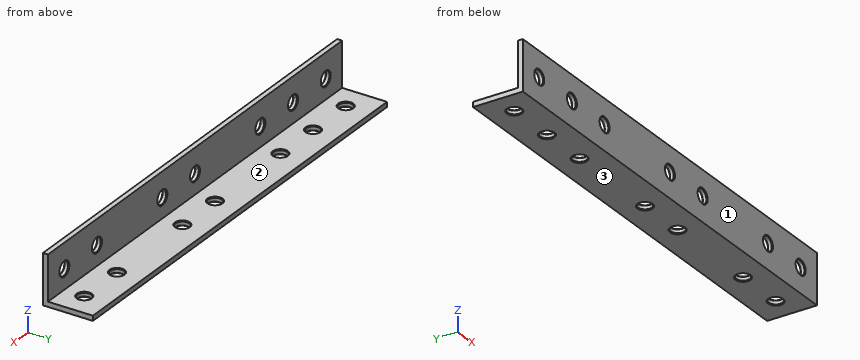
from build123d import *

# Parameters (mm, degrees)
F1_DEPTH = 180
F2_R     = 2.75
F3_DEPTH = 2.001
F4_R     = 2.75
F5_DEPTH = 20.001
F6_SIZE  = 0.3


# Not quite as in the source:
# - a feature names something its author has since deleted; it is built from what else it names


with BuildPart() as f1:
    # F0 (on Right) → F1 (new body)
    with BuildSketch(Plane.YZ):
        Polygon((0, 20), (0, 0), (20, 0), (20, 2), (2, 2), (2, 20), align=None)
    extrude(amount=-F1_DEPTH)

    # F2 (on face) → F3 (cut, through all)
    with BuildSketch(Plane.XY.offset(2)):
        with Locations((-10, 10)):
            Circle(F2_R)
        with Locations((-170, 10)):
            Circle(F2_R)
        with Locations((-150, 10)):
            Circle(F2_R)
        with Locations((-90, 10)):
            Circle(F2_R)
        with Locations((-70, 10)):
            Circle(F2_R)
        with Locations((-30, 10)):
            Circle(F2_R)
        with Locations((-130, 10)):
            Circle(F2_R)
    extrude(amount=-F3_DEPTH, mode=Mode.SUBTRACT)

    # F4 (on face) → F5 (cut, through all)
    with BuildSketch(Plane.XZ):
        with Locations((-170, 10)):
            Circle(F4_R)
        with Locations((-150, 10)):
            Circle(F4_R)
        with Locations((-90, 10)):
            Circle(F4_R)
        with Locations((-70, 10)):
            Circle(F4_R)
        with Locations((-30, 10)):
            Circle(F4_R)
        with Locations((-10, 10)):
            Circle(F4_R)
        with Locations((-130, 10)):
            Circle(F4_R)
    extrude(amount=-F5_DEPTH, mode=Mode.SUBTRACT)

    # F6
    f6_edges = [f1.edges().sort_by_distance(p)[0] for p in [
        (-172.75, 10, 2),
        (-167.25, 10, 1),
        (-172.75, 10, 0),
        (-152.75, 10, 2),
        (-147.25, 10, 1),
        (-152.75, 10, 0),
        (-92.75, 10, 2),
        (-87.25, 10, 1),
        (-92.75, 10, 0),
        (-72.75, 10, 2),
        (-67.25, 10, 1),
        (-72.75, 10, 0),
        (-32.75, 10, 2),
        (-27.25, 10, 1),
        (-32.75, 10, 0),
        (-12.75, 10, 2),
        (-7.25, 10, 1),
        (-12.75, 10, 0),
        (-12.75, 0, 10),
        (-7.25, 1, 10),
        (-12.75, 2, 10),
        (-32.75, 0, 10),
        (-27.25, 1, 10),
        (-32.75, 2, 10),
        (-72.75, 0, 10),
        (-67.25, 1, 10),
        (-72.75, 2, 10),
        (-92.75, 0, 10),
        (-87.25, 1, 10),
        (-92.75, 2, 10),
        (-152.75, 0, 10),
        (-147.25, 1, 10),
        (-152.75, 2, 10),
        (-172.75, 0, 10),
        (-167.25, 1, 10),
        (-172.75, 2, 10),
        (-132.75, 10, 0),
        (-132.75, 10, 2),
        (-132.75, 0, 10),
        (-127.25, 1, 10),
        (-132.75, 2, 10),
    ]]
    chamfer(f6_edges, length=F6_SIZE)


solid = f1.part
Geometry: final body of the model. Coordinates: model frame, mm. Face numbers are marked on the shaded views. Round coordinates to 2 decimals unless told otherwise and drop trailing zeros. Order: outer loops, then holes, each group sorted by start corner. A loop starts at its lowest first (then second) coordinate and runs counter-clockwise, first axis right, second up.
Q1. Section A-A, the plane x = -150. Output: boundary loops of the cut face in (y, z).
Result sheet:
outline: (0, 0) - (6.95, 0) - (7.25, 0.3) - (7.25, 1.7) - (6.95, 2) - (2, 2) - (2, 6.95) - (1.7, 7.25) - (0.3, 7.25) - (0, 6.95) - close; (0, 13.05) - (0.3, 12.75) - (1.7, 12.75) - (2, 13.05) - (2, 20) - (0, 20) - close; (12.75, 0.3) - (13.05, 0) - (20, 0) - (20, 2) - (13.05, 2) - (12.75, 1.7) - close
Q2. Mould query, pull axis Z, two halves, no side actions, for the marked faces 1, 2 and 3. Classes: released by +Z, released by -Z, zero draft, split by the parting line, or undercut.
Result sheet:
face 1: zero draft
face 2: released by +Z
face 3: released by -Z
Q3. Material intervals for probe 1 along Z at (x, y) = (-30, 0.85); probe 2 along Z at (x, y) = (-62, 16.5), sorted ascending.
Result sheet:
probe 1: z = 0 to 7.25, 12.75 to 20
probe 2: z = 0 to 2
Q4. Pin query (flat end, axial travel): pin 1 (3.5 mm diameter, centred on x = -70, y = 10, fed in from +Z); pin 2 (3 mm diameter, centred on x = -75.5, y = 4, fed in from +Z); pin 3 (9 mm diameter, centred on x = -94.5, z = 12.5, fed in from +Y). Return the tip coordinate at first contact, or that it passes through.
Result sheet:
pin 1: passes through
pin 2: stops at z = 2
pin 3: stops at y = 2
Q5. Section D-D, the plane y = 16.5. Output: boundary loops of the cut face in (x, z), and give its area (3 significant figures).
Result sheet:
outline: (-180, 0) - (0, 0) - (0, 2) - (-180, 2) - close
area: 360 mm2
Q6. Section B-B, the plane z = 10. Give the number of separate pieces and of enclosed holes in the cut face, and give its area (3 significant figures).
Result sheet:
separate pieces: 8
enclosed holes: 0
area: 282 mm2
Q7. Section C-C, the plane x = -106. Output: boundary loops of the cut face in (y, z), and give its area (3 significant figures).
Result sheet:
outline: (0, 0) - (20, 0) - (20, 2) - (2, 2) - (2, 20) - (0, 20) - close
area: 76.0 mm2
